For this review, take the finished solid that the model builds, in its own axes (mm). Give positions to 0.01 mm unless a question says otherwise; leave off trailing zeros. Write each loop counter-clockwise with the first axis right and the second up, starting at its lowest first coordinate (ties: lowest second). Pieces come first, ordered by that corner, then holes. Notation, with made-up numbers: (-35, 58) -> (19, 58) arc R9 ccw to (19, 74) -> close; hole circle Ø2 at (-8.75, -15.75). An arc over 180 degrees is marked (long way). Write item = value, one per line.
```python
from build123d import *

# Parameters (mm, degrees)
SKETCH1_R                  = 38.1
BOSS_EXTRUDE1_DEPTH        = 6.35
SKETCH2_R                  = 1.35255
CUT_EXTRUDE1_DEPTH         = 55.254423783
SKETCH3_R                  = 4.7625
CUT_EXTRUDE2_DEPTH         = 6.35
CIRPATTERN2_COUNT          = 3
SKETCH5_R                  = 1.7526
CUT_EXTRUDE4_DEPTH         = 6.35
CIRPATTERN3_COUNT          = 2
F_10_CLEARANCE_HOLE1_D     = 5.1054
F_10_CLEARANCE_HOLE1_DEPTH = 11.43
F_10_CLEARANCE_HOLE1_TIP   = 1.533816902


with BuildPart() as part:
    # Sketch1 → Boss-Extrude1 (new body)
    with BuildSketch(Plane.XY):
        Circle(SKETCH1_R)
    extrude(amount=BOSS_EXTRUDE1_DEPTH)

    # Sketch2 → Cut-Extrude1 (cut, through all)
    with BuildSketch(Plane.XY.offset(6.35)):
        with Locations((0, 23.5585)):
            Circle(SKETCH2_R)
    cut_extrude1 = extrude(amount=-CUT_EXTRUDE1_DEPTH, mode=Mode.SUBTRACT)

    # Sketch3 → Cut-Extrude2 (cut)
    with BuildSketch(Plane(origin=(0, 0, 0), x_dir=(-1, 0, 0), z_dir=(0, 0, -1))):
        Circle(SKETCH3_R)
    extrude(amount=-CUT_EXTRUDE2_DEPTH, mode=Mode.SUBTRACT)

    # CirPattern2: Cut-Extrude1 ×3 about axis
    cirpattern2_axis = Axis((0, 0, 0), (0, 0, 1))
    for i in range(1, CIRPATTERN2_COUNT):
        add(cut_extrude1.rotate(cirpattern2_axis, i * 360 / CIRPATTERN2_COUNT), mode=Mode.SUBTRACT)

    # Sketch5 → Cut-Extrude4 (cut)
    with BuildSketch(Plane(origin=(0, 0, 0), x_dir=(-1, 0, 0), z_dir=(0, 0, -1))):
        with Locations((0, 8.7376)):
            Circle(SKETCH5_R)
    cut_extrude4 = extrude(amount=-CUT_EXTRUDE4_DEPTH, mode=Mode.SUBTRACT)

    # CirPattern3: Cut-Extrude4 ×2 about axis
    cirpattern3_axis = Axis((0, 0, 0), (0, 0, 1))
    for i in range(1, CIRPATTERN3_COUNT):
        add(cut_extrude4.rotate(cirpattern3_axis, i * 360 / CIRPATTERN3_COUNT), mode=Mode.SUBTRACT)

    # 10 Clearance Hole1
    with Locations(Plane(origin=(0, 0, 0), x_dir=(-1, 0, 0), z_dir=(0, 0, -1))):
        with Locations((0, 23.5585), (-20.402259475, -11.77925), (20.402259475, -11.77925)):
            Hole(F_10_CLEARANCE_HOLE1_D / 2, depth=F_10_CLEARANCE_HOLE1_DEPTH)
            with Locations((0, 0, -(F_10_CLEARANCE_HOLE1_DEPTH + F_10_CLEARANCE_HOLE1_TIP / 2))):  # 118° drill point
                Cone(0, F_10_CLEARANCE_HOLE1_D / 2, F_10_CLEARANCE_HOLE1_TIP, mode=Mode.SUBTRACT)


solid = part.part
```
(1) Take a section at A-A (y = 0). Write out the cut boundary in (x, z), plus the area to 3 significant figures.
Answers below:
outline = (-38.1, 0) -> (-4.76, 0) -> (-4.76, 6.35) -> (-38.1, 6.35) -> close; (4.76, 0) -> (38.1, 0) -> (38.1, 6.35) -> (4.76, 6.35) -> close
area = 423 mm^2
(2) Take a section at D-D (x = 19). Write out the cut boundary in (y, z).
Answers below:
outline = (-33.02, 0) -> (-13.91, 0) -> (-13.91, 6.35) -> (-33.02, 6.35) -> close; (-9.65, 0) -> (33.02, 0) -> (33.02, 6.35) -> (-9.65, 6.35) -> close
(3) To check wall thickness, follow probe 1 along Y at (x, z) = (0, 3.75) (1 decimal); probe 2 along Y at (x, z) = (-1.5, 4.5); probe 3 along Y at (x, z) = (21, 4.25). State the ranges of each line that lie inside material, in increasing order.
Answers below:
probe_1 = -38.1 to -10.5, -7 to -4.8, 4.8 to 7, 10.5 to 21, 26.1 to 38.1
probe_2 = -38.07 to -9.64, -7.83 to -4.52, 4.52 to 7.83, 9.64 to 21.49, 25.62 to 38.07
probe_3 = -31.79 to -14.26, -9.3 to 31.79
(4) The part is to be moulded in two halves that separate along X. For faces 1 (the face through (-30.235, -23.183, 3.131)), 2 (the face through (8, 1, 0)), 3 (the face through (-0.809, 7.183, 3.131)), say which applies: released by +X, released by -X, zero draft, split by the parting line, or undercut.
Answers below:
face_1 = split by the parting line
face_2 = zero draft
face_3 = undercut
(5) Take a section at C-C (z = 1.25). Write out the cut boundary in (x, y) (1 decimal).
Answers below:
outline = circle Ø76.2 at (0, 0); hole circle Ø5.1 at (-20.4, -11.8); hole circle Ø9.5 at (0, 0); hole circle Ø5.1 at (0, 23.6); hole circle Ø3.5 at (0, -8.7); hole circle Ø3.5 at (0, 8.7); hole circle Ø5.1 at (20.4, -11.8)
(6) Take a section at B-B (x = 0). Count the separate pieces of the cut face and the enclosed holes in it, plus the area to 3 significant figures.
Answers below:
separate_pieces = 5
enclosed_holes = 0
area = 346 mm^2
(7) For pin 1 (2 mm diameter, centred on y = 9, z = 5, fed in from +X); pin 2 (2 mm diameter, centred on x = 3, z = 4, fed in from +Y); pin 3 (1.5 mm diameter, centred on y = -21.5, z = 4.5, fed in from -X), all flat-tipped, find the tip position at first contact; note any pin that passes through.
Answers below:
pin_1 = 37.25
pin_2 = 38.05
pin_3 = -31.95
